from build123d import *

# Parameters (mm, degrees)
F0_W        = 2
F0_H        = 23
F0_W_2      = 18
F0_R        = 3.5
F1_DEPTH    = 6
F2_DEPTH    = 18
F3_R        = 5
F4_DEPTH    = 25
F5_SIZE2    = 23
F5_SIZE     = 18
F6_T1_DEPTH = 31.7168298797
F6_T3_DEPTH = 32.7168298797
F7_SIZE2    = 2.8562960135
F7_SIZE     = 2


# Not quite as in the source:
# - a fillet or chamfer that OpenCascade refuses, or shapes differently, is made with other operations: its cross-section is extruded or revolved along the edge and cut away or added


with BuildPart() as f1:
    # F0 (on Top) → F1 (new body)
    with BuildSketch(Plane.XY):
        with Locations((-10, -3.5)):
            Rectangle(F0_W, F0_H)
        with Locations((0, -3.5)):
            Rectangle(F0_W_2, F0_H)
        with Locations((0, -5)):
            Circle(F0_R, mode=Mode.SUBTRACT)
        with Locations((10, -3.5)):
            Rectangle(F0_W, F0_H)
        Polygon((9, 8), (11, 8), (11, 15), (-11, 15), (-11, 8), (-9, 8), align=None)
    extrude(amount=-F1_DEPTH)

    # F0 (on Top) → F2 (join)
    with BuildSketch(Plane.XY):
        Polygon((9, 8), (11, 8), (11, 15), (-11, 15), (-11, 8), (-9, 8), align=None)
        with Locations((-10, -3.5)):
            Rectangle(F0_W, F0_H)
        with Locations((10, -3.5)):
            Rectangle(F0_W, F0_H)
    extrude(amount=F2_DEPTH)

    # F3 (on face) → F4 (cut)
    with BuildSketch(Plane.XZ.offset(-8)):
        with Locations((0, 9)):
            Circle(F3_R)
    extrude(amount=-F4_DEPTH, mode=Mode.SUBTRACT)

    # F5
    f5_edges = [f1.edges().sort_by_distance(p)[0] for p in [
        (-10, -15, 18),
        (10, -15, 18),
    ]]
    f5_side = f1.faces().sort_by_distance((0, -15, -5.674424))[0]
    chamfer(f5_edges, length=F5_SIZE, length2=F5_SIZE2, reference=f5_side)

    # F6: chamfer of 5 on 4 edges, made by hand

    # F6_s2 → F6_t1 (cut)
    with BuildSketch(Plane.XY.offset(-18.8584149398)):
        Polygon((6, -15), (11, -10), (11, -15), align=None)
        Polygon((-6, -15), (-11, -10), (-11, -15), align=None)
    extrude(amount=F6_T1_DEPTH, mode=Mode.SUBTRACT)

    # F6_s4 → F6_t3 (cut)
    with BuildSketch(Plane.XZ.offset(-27.8584149398)):
        Polygon((11, 13), (6, 18), (11, 18), align=None)
        Polygon((-11, 13), (-6, 18), (-11, 18), align=None)
    extrude(amount=F6_T3_DEPTH, mode=Mode.SUBTRACT)

    # F7
    f7_edges = [f1.edges().sort_by_distance(p)[0] for p in [
        (-3.5, -5, 0),
    ]]
    f7_side = f1.faces().sort_by_distance((-3.5, -5, -3))[0]
    chamfer(f7_edges, length=F7_SIZE, length2=F7_SIZE2, reference=f7_side)


solid = f1.part
Model file for the job. Use its own axes, mm. A direction names the side the tool comes from. Give positions to 0.01 mm unless a question says otherwise; leave off trailing zeros. Order: outer loops, then holes, each group sorted by start corner. A loop starts at its lowest first (then second) coordinate and runs counter-clockwise, first axis right, second up. Notation, with made-up numbers: (87, 63) - (112, 63) arc R24 ccw to (112, 92) - close; hole circle Ø9 at (14.5, 34). An arc over 180 degrees is marked (long way). Write item = value, one per line. Start each with the question number.
1. Drop flat-ended pins along their axis: P1, Ø2, axis at x = -4, y = -2, coming from the +Z side; P2, Ø5, axis at x = 2.5, z = 8.5, coming from the -Y side; P3, Ø9, axis at x = -3.5, y = -1.5, coming from the +Z side. Give the stop position or say it passes through.
2. Cut at C-C, the plane x = 0. List the corners of the cut face in (y, z).
3. Cut at D-D, the plane z = -2.5. List the corners of the cut face in (x, y), and give its area (3 significant figures).
4. Cut at A-A, the plane z = 9. List the corners of the cut face in (x, y), and give its area (3 significant figures).
5. Cut at B-B, the plane y = 8.5. List the corners of the cut face in (x, z), and give its area (3 significant figures).
6. Which spindle directions (+Z, -Z, +X, -X, +Y, -Y) get a long thin tool onto all of the face, cutting with end or side? Do faces 4 (the flat face through (0, -15, -3)), 5 (the flat face through (-9, 0, 6)). Say none if no direction does.
7. Two-plate mould, pull along X, no slides. Class faces 1 (the flat face through (11, 2, 3)), 2 (the flat face through (9, 0, 6)), 3 (the flat face through (-9, 10, 15)): pulls with the +X half, pulls with the -X half, needs draft (parallel to the pull), parting line crosses it, or undercut.
8. Probe line 1 along Y through (x, z) = (0, -2.85); line 2 along X through (y, z) = (-8.25, 4); line 3 along Z through (x, y) = (0, 12.5). List the from-to ranges inside material, lowest first.
Taken from the geometry:
q1.P1 = -0.25
q1.P2 = 8
q1.P3 = 0
q2.outline = (-15, -6) - (-8.5, -6) - (-8.5, -2) - (-11.36, 0) - (-15, 0) - close; (-1.5, -6) - (15, -6) - (15, 4) - (8, 4) - (8, 0) - (1.36, 0) - (-1.5, -2) - close; (8, 14) - (15, 14) - (15, 18) - (8, 18) - close
q3.outline = (-11, -10) - (-6, -15) - (6, -15) - (11, -10) - (11, 15) - (-11, 15) - close; hole circle Ø7 at (0, -5)
q3.area = 597 mm²
q4.outline = (-11, -3.5) - (-9, -3.5) - (-9, 8) - (-5, 8) - (-5, 15) - (-11, 15) - close; (5, 8) - (9, 8) - (9, -3.5) - (11, -3.5) - (11, 15) - (5, 15) - close
q4.area = 130 mm²
q5.outline = (-11, -6) - (11, -6) - (11, 13) - (6, 18) - (-6, 18) - (-11, 13) - close; hole circle Ø10 at (0, 9)
q5.area = 424 mm²
q6.face_4 = +Z, -Z, +X, -X, -Y
q6.face_5 = +Z, -Y
q7.face_1 = pulls with the +X half
q7.face_2 = undercut
q7.face_3 = pulls with the -X half
q8.line_1 = -15 to -8.5, -1.5 to 15
q8.line_2 = -11 to -9, 9 to 11
q8.line_3 = -6 to 4, 14 to 18
